from build123d import *

# Parameters (mm, degrees)
SKETCH1_W           = 50.8
SKETCH1_H           = 25.4
SKETCH1_W_2         = 44.45
SKETCH1_H_2         = 19.05
BOSS_EXTRUDE1_DEPTH = 304.8
SKETCH2_R           = 4.7625
CUT_EXTRUDE1_DEPTH  = 307.909367729
SKETCH3_R           = 3.175
CUT_EXTRUDE2_DEPTH  = 310.265209812
SKETCH4_W           = 50.8
SKETCH4_H           = 25.4
CUT_EXTRUDE3_DEPTH  = 88.9


with BuildPart() as part:
    # Sketch1 → Boss-Extrude1 (new body)
    with BuildSketch(Plane.XY):
        Rectangle(SKETCH1_W, SKETCH1_H)
        Rectangle(SKETCH1_W_2, SKETCH1_H_2, mode=Mode.SUBTRACT)
    extrude(amount=BOSS_EXTRUDE1_DEPTH)

    # Sketch2 → Cut-Extrude1 (cut, through all)
    with BuildSketch(Plane(origin=(0, 12.7, 0), x_dir=(1, 0, 0), z_dir=(0, 1, 0))):
        with Locations(Location((0, -285.75, 0), (0, 0, 270))):
            Circle(SKETCH2_R)
    extrude(amount=-CUT_EXTRUDE1_DEPTH, mode=Mode.SUBTRACT)

    # Sketch3 → Cut-Extrude2 (cut, through all)
    with BuildSketch(Plane.ZY.offset(25.4)):
        with Locations((109.947638526, -1.739817444)):
            Circle(SKETCH3_R)
    extrude(amount=-CUT_EXTRUDE2_DEPTH, mode=Mode.SUBTRACT)

    # Sketch4 → Cut-Extrude3 (cut)
    with BuildSketch(Plane(origin=(0, 0, 0), x_dir=(-1, 0, 0), z_dir=(0, 0, -1))):
        Rectangle(SKETCH4_W, SKETCH4_H)
    extrude(amount=-CUT_EXTRUDE3_DEPTH, mode=Mode.SUBTRACT)


solid = part.part
Source: CAD feature listing. Evaluate the final solid. Frame: model axes, mm. A direction names the side the tool comes from. Give positions to 0.01 mm unless a question says otherwise; leave off trailing zeros. Loops run counter-clockwise (first coordinate to the right, second up) from the corner with the lowest first, then second, coordinate; pieces in that order, holes last. Notation, with made-up numbers: (8, 53) -> (25, 53) arc R28 cw to (25, 85) -> close; hole circle Ø3 at (77, 67). An arc over 180 degrees is marked (long way). Use a Markdown table: item, result. Add a question column.
1) Pull-direction query (X, two-part tool) for faces 1 (the face through (25.4, 0, 195)), 2 (the face through (-25.4, 0, 195)), 3 (the face through (0, -9.525, 195)), 4 (the face through (0, 10, 88.9)); classes: +X half, -X half, draft (parallel to the pull), parting line (faces both ways), or undercut.
2) Section query A-A, the plane z = 285.75. Return the cut outline in (x, y) (1 decimal).
3) Section query D-D, the plane x = 0. Return the cut outline in (y, z) (1 decimal).
4) Section query C-C, the plane z = 174.5. Return the cut outline in (x, y) (3 decimals).
5) Line query: line 1 along Y through (x, z) = (-19.5, 281) (3 decimals); line 2 along X through (y, z) = (8.25, 185) (3 decimals); line 3 along X through (y, z) = (-11.3, 285.75). Output: solid intervals per line, ascending. Write a range as [from, to].
6) Reachability of faces 5 (the face through (0.209, -11.09, 280.992)), 6 (the face through (0, 9.525, 195)) from +Z, -Z, +X, -X, +Y, -Y: full face, straight path, thin tool, end or side. Return the list, or none.
7) Section query B-B, the plane x = -17. Return the cut outline in (y, z) (3 decimals), then the cut area to 3 significant figures.
Numbers:
| question | item | result |
|---|---|---|
| 1 | face 1 | +X half |
| 1 | face 2 | -X half |
| 1 | face 3 | undercut |
| 1 | face 4 | draft |
| 2 | outline | (-25.4, -12.7) -> (-4.8, -12.7) -> (-4.8, -9.5) -> (-22.2, -9.5) -> (-22.2, 9.5) -> (-4.8, 9.5) -> (-4.8, 12.7) -> (-25.4, 12.7) -> close; (4.8, -12.7) -> (25.4, -12.7) -> (25.4, 12.7) -> (4.8, 12.7) -> (4.8, 9.5) -> (22.2, 9.5) -> (22.2, -9.5) -> (4.8, -9.5) -> close |
| 3 | outline | (-12.7, 88.9) -> (-9.5, 88.9) -> (-9.5, 281) -> (-12.7, 281) -> close; (-12.7, 290.5) -> (-9.5, 290.5) -> (-9.5, 304.8) -> (-12.7, 304.8) -> close; (9.5, 88.9) -> (12.7, 88.9) -> (12.7, 281) -> (9.5, 281) -> close; (9.5, 290.5) -> (12.7, 290.5) -> (12.7, 304.8) -> (9.5, 304.8) -> close |
| 4 | outline | (-25.4, -12.7) -> (25.4, -12.7) -> (25.4, 12.7) -> (-25.4, 12.7) -> close; hole (-22.225, -9.525) -> (22.225, -9.525) -> (22.225, 9.525) -> (-22.225, 9.525) -> close |
| 5 | line 1 | y = [-12.7, -9.525], [9.525, 12.7] |
| 5 | line 2 | x = [-25.4, -22.225], [22.225, 25.4] |
| 5 | line 3 | x = [-25.4, -4.76], [4.76, 25.4] |
| 6 | face 5 | +Y, -Y |
| 6 | face 6 | +Z, -Z |
| 7 | outline | (-12.7, 88.9) -> (-9.525, 88.9) -> (-9.525, 304.8) -> (-12.7, 304.8) -> close; (9.525, 88.9) -> (12.7, 88.9) -> (12.7, 304.8) -> (9.525, 304.8) -> close |
| 7 | area | 1,370 mm2 |
